Here's how the part is built. I have some questions about the finished solid (model axes, mm). Face numbers are marked on the shaded views. A direction names the side the tool comes from. Coordinates: 2 decimals unless noted, no trailing zeros. Loops run counter-clockwise (first coordinate to the right, second up) from the corner with the lowest first, then second, coordinate; pieces in that order, holes last. Notation, with made-up numbers: M 71,-15.75 L 124,-15.75 A22 ccw 124,3.25 Z; hole C 63,38 d4. An arc over 180 degrees is marked long. Use CSV: the item, a comma, the result in double quotes. Start each with the question number.
Q1. Which directions (+Z, -Z, +X, -X, +Y, -Y) give clear straight access to the entire face, cutting with the end or side of a thin tool? Please do the marked faces 1 and 2.
Q2. If we section it at B-B (x = 31): Please give me the cut outline in (y, z), and give its area (3 significant figures).
Q3. Please list where these lines run through material, in increasing order: probe 1 along X at (y, z) = (66, 2); probe 2 along X at (y, z) = (49, 15.5); probe 3 along X at (y, z) = (54, 13.75). Write a range as [from, to].
Q4. For pin 1 Ø4 at (x, y) = (42.5, 67) entering from +Z; pin 2 Ø5 at (y, z) = (60.5, 19.5) entering from +X; pin 3 Ø1 at (y, z) = (38, 16) entering from -X; pin 4 Ø1.5 at (x, z) = (-59.5, 21) entering from -Y, each with a flat end and sliding along its axis, tell me the tip position at first contact or that it passes through.
Q5. If we mould it in two halves opening along X, with no side actions, what happens to the marked faces 3, 4 and 5? For each: +X half, -X half, draft (parallel to the pull), parting line (faces both ways), or undercut.
Q6. If we section it at C-C (x = 79.5): Please give me the cut outline in (y, z), and give its area (3 significant figures).
Q7. If we section it at A-A (z = 19): Please give me the cut outline in (x, y).
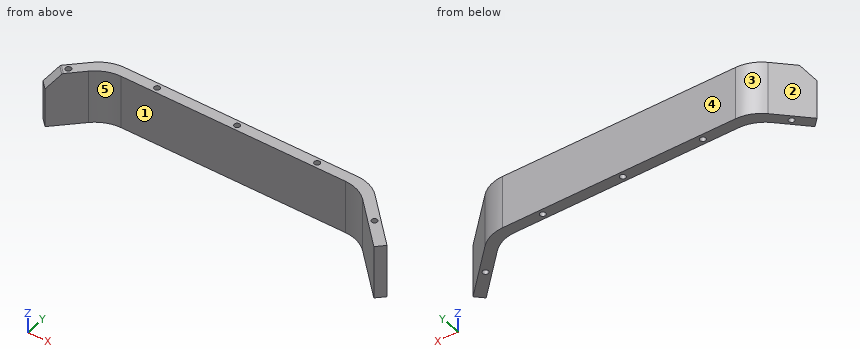
Solid Edge part; units mm, degrees
sketch "Sketch1" plane through (0, 0, 0) normal (0, 0, 1) x (1, 0, 0)
  line L0 (-65.4804, 64) -> (60.4804, 64)
  arc A0 (60.4804, 64) -> (74.6226, 58.1421) centre (60.4804, 44) cw
  line L1 (98.6495, 34.1152) -> (74.6226, 58.1421)
  line L2 (102.8921, 38.3579) -> (98.6495, 34.1152)
  line L3 (77.1079, 64.1421) -> (102.8921, 38.3579)
  arc A1 (62.9657, 70) -> (77.1079, 64.1421) centre (62.9657, 50) cw
  line L4 (62.9657, 70) -> (-67.9657, 70)
  arc A2 (-82.1079, 64.1421) -> (-67.9657, 70) centre (-67.9657, 50) cw
  line L5 (-82.1079, 64.1421) -> (-97.8921, 48.3579)
  line L6 (-97.8921, 48.3579) -> (-93.6495, 44.1152)
  line L7 (-93.6495, 44.1152) -> (-79.6226, 58.1421)
  arc A3 (-79.6226, 58.1421) -> (-65.4804, 64) centre (-65.4804, 44) cw
  circle A4 centre (-47.5, 67) radius 1.6
  circle A5 centre (-87.8787, 54.1287) radius 1.6
  circle A6 centre (-2.5, 67) radius 1.6
  circle A7 centre (42.5, 67) radius 1.6
  circle A8 centre (87.8787, 49.1287) radius 1.6
extrude "Protrusion1" add sketch "Sketch1" along normal blind 30
chamfer "Chamfer_1" distance 8 angle 45 1 edges at (-95.7708, 46.2365, 30) measured on face at (-66.4359, 64.378, 30)
fillet "Round_7" radius 1 1 edges at (-90.114, 51.8934, 30)
Results below:
1,face 1,"+Z, -Z, -Y"
1,face 2,"+Z, -Z, -X, +Y"
2,outline,"M 64,0 L 70,0 L 70,30 L 64,30 Z"
2,area,"180 mm^2"
3,probe 1,"[-79.97, -48.75], [-46.25, -3.75], [-1.25, 41.25], [43.75, 74.97]"
3,probe 2,"[-97.25, -88.76], [83.76, 86.28], [89.47, 92.25]"
3,probe 3,"[-92.25, -89.47], [-86.28, -83.76], [78.76, 87.25]"
4,pin 1,"z = 30"
4,pin 2,"x = 83.25"
4,pin 3,"x = 94.26"
4,pin 4,"y = 64"
5,face 3,"-X half"
5,face 4,"draft"
5,face 5,"undercut"
6,outline,"M 53.26,0 L 61.75,0 L 61.75,30 L 53.26,30 Z"
6,area,"255 mm^2"
7,outline,"M -97.89,48.36 L -93.65,44.12 L -79.62,58.14 A20 cw -65.48,64 L 60.48,64 A20 cw 74.62,58.14 L 98.65,34.12 L 102.89,38.36 L 77.11,64.14 A20 ccw 62.97,70 L -67.97,70 A20 ccw -82.11,64.14 Z; hole C -87.88,54.13 d3.2; hole C -47.5,67 d3.2; hole C -2.5,67 d3.2; hole C 42.5,67 d3.2; hole C 87.88,49.13 d3.2"
